Check sheet for the drawn part. Datum: minimum x, y, z corner. Units: mm. A direction names the side the tool comes from. Give positions to 0.01 mm unless a question says otherwise; leave off trailing zeros. Order: outer loops, then holes, each group sorted by start corner. A loop starts at its lowest first (then second) coordinate and runs counter-clockwise, first axis right, second up. Notation, with made-up numbers: (-26, 65.5) -> (-4, 65.5) arc R23 ccw to (-4, 76.5) -> close; hole circle Ø9 at (49.25, -21). An arc over 180 degrees is marked (long way). Return JSON: item names as keys, results as strings. Group by question number.
(1) Cross-section at B-B on z = 22.5. State how many separate pieces and enclosed holes the cut face has, then the cut area to 3 significant figures.
(2) Release check for a two-part mould opening along Y. For the marked faces 3, 4 and 5 record: pulls with the +Y half, pulls with the -Y half, needs draft (parallel to the pull), parting line crosses it, or undercut.
(3) Cross-section at C-C on y = 105. Enter the section's corners in (x, z).
(4) Cross-section at A-A on x = 105. Enter the section's corners in (y, z), then the cut area to 3 significant figures.
(5) Thickness scan on line 1 along Y through (x, z) = (86.5, 38.5) (1 decimal); line 2 along Y through (x, z) = (87.5, 31) (1 decimal); line 3 along X through (y, z) = (231, 10) (1 decimal). Record the ranges inside material, lowest first.
(6) Depth check by flat-ended pin: pin 1 Ø1 at (y, z) = (235.5, 10) entering from -X; pin 2 Ø10 at (x, z) = (26.5, 49.5) entering from +Y; pin 3 Ø5 at (y, z) = (254.5, 38) entering from +X (1 decimal). Enter the tip coordinate at first touch or a pass-through.
(7) Tool access check on the marked faces 1 and 2. Record the directions out of +Z, -Z, +X, -X, +Y, -Y that give a thin tool (end or side, any length) a straight path to the whole face; none if there is none.
(8) Cross-section at D-D on y = 245. Enter the section's corners in (x, z), then the cut area to 3 significant figures.
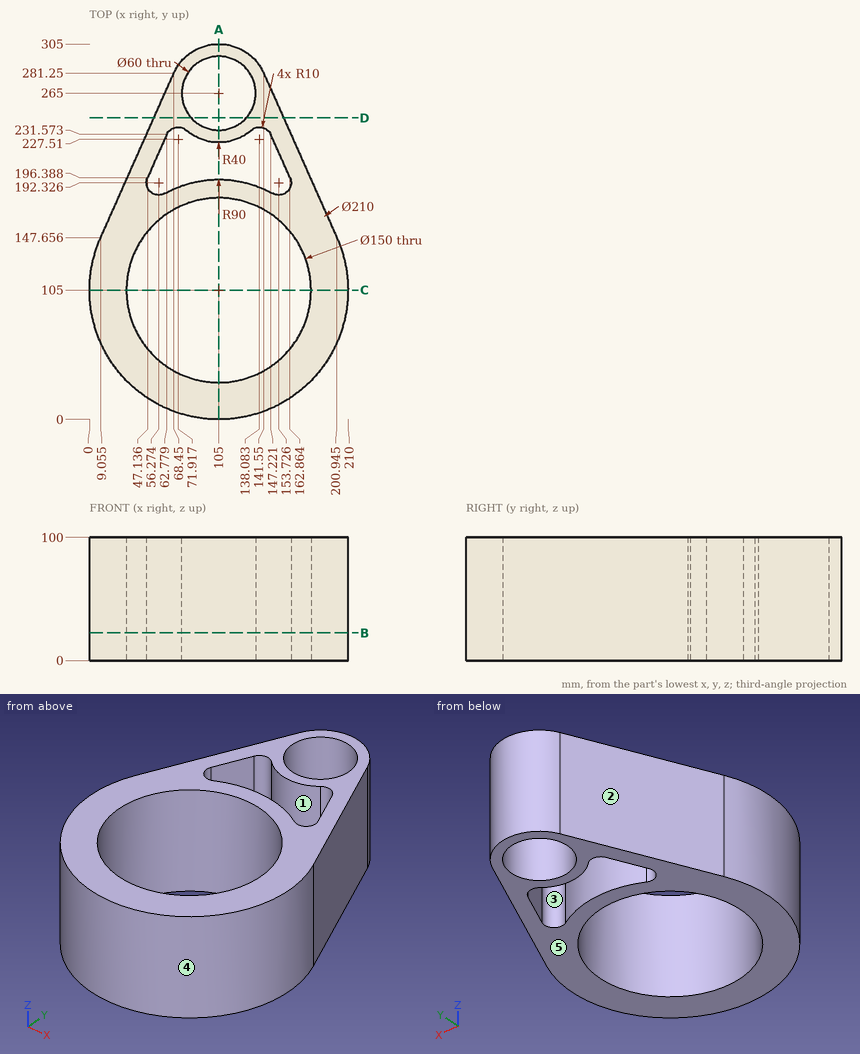
Verdict:
{
 "1": {"separate pieces": "1", "enclosed holes": "3", "area": "20,200 mm²"},
 "2": {"face 3": "undercut", "face 4": "parting line crosses it", "face 5": "needs draft"},
 "3": {"outline": "(0, 0) -> (30, 0) -> (30, 100) -> (0, 100) -> close; (180, 0) -> (210, 0) -> (210, 100) -> (180, 100) -> close"},
 "4": {"outline": "(0, 0) -> (30, 0) -> (30, 100) -> (0, 100) -> close; (180, 0) -> (195, 0) -> (195, 100) -> (180, 100) -> close; (225, 0) -> (235, 0) -> (235, 100) -> (225, 100) -> close; (295, 0) -> (305, 0) -> (305, 100) -> (295, 100) -> close", "area": "6,500 mm²"},
 "5": {"line 1": "1.6 to 32.3, 177.7 to 193.1, 229.5 to 241.4, 288.6 to 300.5", "line 2": "1.5 to 32.1, 177.9 to 193.3, 229 to 240.6, 289.4 to 301", "line 3": "46.1 to 62.5, 83.9 to 126.1, 147.5 to 163.9"},
 "6": {"pin 1": "x = 47.89", "pin 2": "y = 198.14", "pin 3": "x = 154.6"},
 "7": {"face 1": "+Z, -Z", "face 2": "+Z, -Z, -X, +Y"},
 "8": {"outline": "(52.33, 0) -> (82.64, 0) -> (82.64, 100) -> (52.33, 100) -> close; (127.36, 0) -> (157.67, 0) -> (157.67, 100) -> (127.36, 100) -> close", "area": "6,060 mm²"}
}
